from build123d import *

# Parameters (mm, degrees)
BOSS_EXTRUDE1_DEPTH   = 12.446
F_6_CLEARANCE_HOLE1_D = 4.134
CHAMFER1_SIZE         = 0.433
FILLET1_R             = 0.381


with BuildPart() as part:
    # Sketch1 → Boss-Extrude1 (new body)
    with BuildSketch(Plane.XY.offset(5.08)):
        Polygon((5.4737, 4.3434), (-5.4737, 4.3434), (-5.4737, 2.38887), (-3.08483, 0), (3.08483, 0), (5.4737, 2.38887), align=None)
    extrude(amount=-BOSS_EXTRUDE1_DEPTH)

    # #6 Clearance Hole1 (through all)
    with Locations(Plane(origin=(0, 4.3434, 0), x_dir=(1, 0, 0), z_dir=(0, 1, 0))):
        with Locations((0, 0)):
            Hole(F_6_CLEARANCE_HOLE1_D / 2)

    # Chamfer1
    chamfer1_edges = [part.edges().sort_by_distance(p)[0] for p in [
        (2.067, 4.3434, 0),
        (2.067, 0, 0),
    ]]
    chamfer(chamfer1_edges, length=CHAMFER1_SIZE)

    # Fillet1
    fillet1_edges = [part.edges().sort_by_distance(p)[0] for p in [
        (5.4737, 2.38887, -1.143),
        (3.08483, 0, -1.143),
        (-3.08483, 0, -1.143),
        (-5.4737, 2.38887, -1.143),
        (-5.4737, 4.3434, -1.143),
        (5.4737, 4.3434, -1.143),
    ]]
    fillet(fillet1_edges, radius=FILLET1_R)


solid = part.part
For this review, take the finished solid that the model builds, in its own axes (mm). Round coordinates to 2 decimals unless told otherwise and drop trailing zeros. Loops run counter-clockwise (first coordinate to the right, second up) from the corner with the lowest first, then second, coordinate; pieces in that order, holes last. Notation, with made-up numbers: (25.25, 35.25) - (36.25, 35.25) arc R9 cw to (36.25, 43.25) - close; hole circle Ø7 at (-23.5, 37). An arc over 180 degrees is marked (long way). One line per question, with ' | ' between items.
Q1. Take a section at C-C (y = 2.7). Give the boundary of the cut face in (x, z).
Taken from the geometry:
outline: (-5.47, -7.37) - (5.47, -7.37) - (5.47, 5.08) - (-5.47, 5.08) - close; hole circle Ø4.13 at (0, 0)
Q2. Take a section at A-A (z = 0). Give the boundary of the cut face in (x, y).
Taken from the geometry:
outline: (-5.47, 2.55) arc R0.38 ccw to (-5.36, 2.28) - (-3.2, 0.11) arc R0.38 ccw to (-2.93, 0) - (-2.5, 0) - (-2.07, 0.43) - (-2.07, 3.91) - (-2.5, 4.34) - (-5.09, 4.34) arc R0.38 ccw to (-5.47, 3.96) - close; (2.07, 0.43) - (2.5, 0) - (2.93, 0) arc R0.38 ccw to (3.2, 0.11) - (5.36, 2.28) arc R0.38 ccw to (5.47, 2.55) - (5.47, 3.96) arc R0.38 ccw to (5.09, 4.34) - (2.5, 4.34) - (2.07, 3.91) - close
Q3. Take a section at B-B (x = 0). Give the boundary of the cut face in (y, z).
Taken from the geometry:
outline: (0, -7.37) - (4.34, -7.37) - (4.34, -2.5) - (3.91, -2.07) - (0.43, -2.07) - (0, -2.5) - close; (0, 2.5) - (0.43, 2.07) - (3.91, 2.07) - (4.34, 2.5) - (4.34, 5.08) - (0, 5.08) - close
Q4. For line 1 along X through (y, z) = (3.15, 0); line 2 along Z through (x, y) = (0, 1.6); line 3 along X through (y, z) = (2.4, 0), list the stretches that pass through material, from the lowest coordinate up. Write a range as [from, to].
Taken from the geometry:
line 1: x = [-5.47, -2.07], [2.07, 5.47] | line 2: z = [-7.37, -2.07], [2.07, 5.08] | line 3: x = [-5.44, -2.07], [2.07, 5.44]
Q5. Take a section at D-D (z = -5). Give the boundary of the cut face in (x, y), and give its area (3 significant figures).
Taken from the geometry:
outline: (-5.47, 2.55) arc R0.38 ccw to (-5.36, 2.28) - (-3.2, 0.11) arc R0.38 ccw to (-2.93, 0) - (2.93, 0) arc R0.38 ccw to (3.2, 0.11) - (5.36, 2.28) arc R0.38 ccw to (5.47, 2.55) - (5.47, 3.96) arc R0.38 ccw to (5.09, 4.34) - (-5.09, 4.34) arc R0.38 ccw to (-5.47, 3.96) - close | area: 41.8 mm²
Q6. The part is to be moulded in two halves that separate along Z. For faces 1 (the flat face through (0, 2, 5.08)), 2 (the cylindrical face through (1.64, 2.15, 1.26)), 3 (the flat face through (-4.294, 1.21, -1.056)), say which applies: released by +Z, released by -Z, zero draft, split by the parting line, or undercut.
Taken from the geometry:
face 1: released by +Z | face 2: undercut | face 3: zero draft
